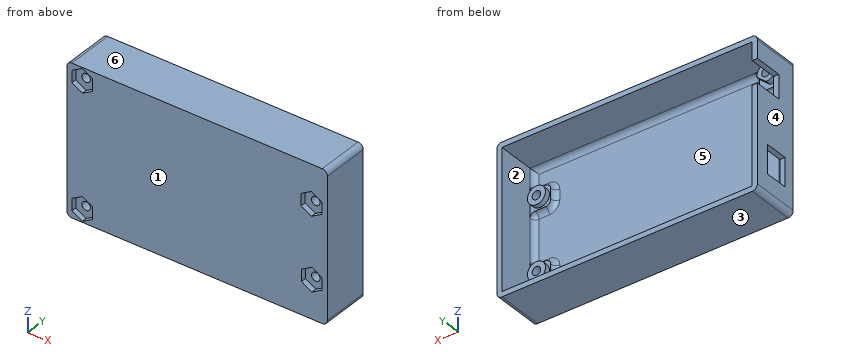
from build123d import *

# Parameters (mm, degrees)
SKETCH1_W           = 100.75
SKETCH1_H           = 57.75
SKETCH1_W_2         = 96.75
SKETCH1_H_2         = 53.75
SKETCH1_R           = 1.65
BOSS_EXTRUDE1_DEPTH = 2
SKETCH2_R           = 3.5
SKETCH2_R_2         = 1.65
BOSS_EXTRUDE2_DEPTH = 4
SKETCH3_W           = 100.75
SKETCH3_H           = 57.75
SKETCH3_W_2         = 96.75
SKETCH3_H_2         = 53.75
BOSS_EXTRUDE3_DEPTH = 16.4
FILLET1_R           = 2
SKETCH5_W           = 8
SKETCH5_H           = 8
SKETCH5_R           = 1.65
BOSS_EXTRUDE4_DEPTH = 2
FILLET3_R           = 2
FILLET4_R           = 2
SKETCH6_W           = 9.2
SKETCH6_H           = 11
SKETCH6_W_2         = 8
SKETCH6_H_2         = 2.6
CUT_EXTRUDE2_DEPTH  = 2
CUT_EXTRUDE3_DEPTH  = 2


with BuildPart() as part:
    # Sketch1 → Boss-Extrude1 (new body)
    # profile 1 of 2: a face of its own
    with BuildSketch(Plane(origin=(0, 0, 0), x_dir=(1, 0, 0), z_dir=(0, 1, 0))):
        with Locations((0.125, -0.125)):
            Rectangle(SKETCH1_W, SKETCH1_H)
        with Locations((0.125, -0.125)):
            Rectangle(SKETCH1_W_2, SKETCH1_H_2, mode=Mode.SUBTRACT)
    # profile 2 of 2: a face of its own
    with BuildSketch(Plane(origin=(0, 0, 0), x_dir=(1, 0, 0), z_dir=(0, 1, 0))):
        with Locations((0.125, -0.125)):
            Rectangle(SKETCH1_W_2, SKETCH1_H_2)
        with Locations(Location((-44.25, -24, 0), (0, 0, 270))):
            Circle(SKETCH1_R, mode=Mode.SUBTRACT)
        with Locations(Location((-44.25, 23.75, 0), (0, 0, 270))):
            Circle(SKETCH1_R, mode=Mode.SUBTRACT)
        with Locations(Location((44.5, 14, 0), (0, 0, 270))):
            Circle(SKETCH1_R, mode=Mode.SUBTRACT)
        with Locations(Location((44.5, -14.25, 0), (0, 0, 270))):
            Circle(SKETCH1_R, mode=Mode.SUBTRACT)
    extrude(amount=BOSS_EXTRUDE1_DEPTH)

    # Sketch2 → Boss-Extrude2 (add)
    # profile 1 of 4: a face of its own
    with BuildSketch(Plane(origin=(0, 2, 0), x_dir=(1, 0, 0), z_dir=(0, 1, 0))):
        with Locations(Location((44.5, 14, 0), (0, 0, 270))):
            Circle(SKETCH2_R)
        with Locations(Location((44.5, 14, 0), (0, 0, 270))):
            Circle(SKETCH2_R_2, mode=Mode.SUBTRACT)
    # profile 2 of 4: a face of its own
    with BuildSketch(Plane(origin=(0, 2, 0), x_dir=(1, 0, 0), z_dir=(0, 1, 0))):
        with Locations(Location((44.5, -14.25, 0), (0, 0, 270))):
            Circle(SKETCH2_R)
        with Locations(Location((44.5, -14.25, 0), (0, 0, 270))):
            Circle(SKETCH2_R_2, mode=Mode.SUBTRACT)
    # profile 3 of 4: a face of its own
    with BuildSketch(Plane(origin=(0, 2, 0), x_dir=(1, 0, 0), z_dir=(0, 1, 0))):
        with BuildLine():
            Line((-44.303434376, -20.500407914), (-40.787920243, -23.486187041))
            ThreePointArc((-40.787920243, -23.486187041), (-41.085130973, -25.494524687), (-42.447224362, -27))
            Line((-42.447224362, -27), (-46.052775638, -27))
            ThreePointArc((-46.052775638, -27), (-47.629726797, -23.090358985), (-44.303434376, -20.500407914))
        make_face()
        with Locations(Location((-44.25, -24, 0), (0, 0, 270))):
            Circle(SKETCH2_R_2, mode=Mode.SUBTRACT)
    # profile 4 of 4: a face of its own
    with BuildSketch(Plane(origin=(0, 2, 0), x_dir=(1, 0, 0), z_dir=(0, 1, 0))):
        with BuildLine():
            Line((-46.052775638, 26.75), (-42.447224362, 26.75))
            ThreePointArc((-42.447224362, 26.75), (-44.25, 20.25), (-46.052775638, 26.75))
        make_face()
        with Locations(Location((-44.25, 23.75, 0), (0, 0, 270))):
            Circle(SKETCH2_R_2, mode=Mode.SUBTRACT)
    extrude(amount=BOSS_EXTRUDE2_DEPTH)

    # Sketch3 → Boss-Extrude3 (add)
    with BuildSketch(Plane(origin=(0, 2, 0), x_dir=(1, 0, 0), z_dir=(0, 1, 0))):
        with Locations((0.125, -0.125)):
            Rectangle(SKETCH3_W, SKETCH3_H)
        with Locations((0.125, -0.125)):
            Rectangle(SKETCH3_W_2, SKETCH3_H_2, mode=Mode.SUBTRACT)
    extrude(amount=BOSS_EXTRUDE3_DEPTH)

    # Fillet1
    fillet1_edges = [part.edges().sort_by_distance(p)[0] for p in [
        (50.5, 9.2, 29),
        (-50.25, 9.2, 29),
        (-50.25, 9.2, -28.75),
        (50.5, 9.2, -28.75),
    ]]
    fillet(fillet1_edges, radius=FILLET1_R)

    # Sketch5 → Boss-Extrude4 (add)
    # profile 1 of 4: a face of its own
    with BuildSketch(Plane(origin=(0, 2, 0), x_dir=(1, 0, 0), z_dir=(0, 1, 0))):
        with Locations((44.5, 14)):
            Rectangle(SKETCH5_W, SKETCH5_H)
        with Locations(Location((44.5, 14, 0), (0, 0, 270))):
            Circle(SKETCH5_R, mode=Mode.SUBTRACT)
    # profile 2 of 4: a face of its own
    with BuildSketch(Plane(origin=(0, 2, 0), x_dir=(1, 0, 0), z_dir=(0, 1, 0))):
        with Locations((44.5, -14.25)):
            Rectangle(SKETCH5_W, SKETCH5_H)
        with Locations(Location((44.5, -14.25, 0), (0, 0, 270))):
            Circle(SKETCH5_R, mode=Mode.SUBTRACT)
    # profile 3 of 4: a face of its own
    with BuildSketch(Plane(origin=(0, 2, 0), x_dir=(1, 0, 0), z_dir=(0, 1, 0))):
        with Locations((-44.25, -23)):
            Rectangle(SKETCH5_W, SKETCH5_H)
        with Locations(Location((-44.25, -24, 0), (0, 0, 270))):
            Circle(SKETCH5_R, mode=Mode.SUBTRACT)
    # profile 4 of 4: a face of its own
    with BuildSketch(Plane(origin=(0, 2, 0), x_dir=(1, 0, 0), z_dir=(0, 1, 0))):
        with Locations((-44.25, 22.75)):
            Rectangle(SKETCH5_W, SKETCH5_H)
        with Locations(Location((-44.25, 23.75, 0), (0, 0, 270))):
            Circle(SKETCH5_R, mode=Mode.SUBTRACT)
    extrude(amount=BOSS_EXTRUDE4_DEPTH)

    # Fillet3
    fillet3_edges = [part.edges().sort_by_distance(p)[0] for p in [
        (40.5, 3, -18),
        (40.5, 3, -10),
        (48.5, 3, -10),
        (48.5, 3, -18),
        (40.5, 3, 10.25),
        (40.5, 3, 18.25),
        (48.5, 3, 18.25),
        (48.5, 3, 10.25),
        (-48.25, 3, 19),
        (-40.25, 3, 27),
        (-40.25, 3, 19),
        (-40.25, 3, -26.75),
        (-48.25, 3, -18.75),
        (-40.25, 3, -18.75),
    ]]
    fillet(fillet3_edges, radius=FILLET3_R)

    # Fillet4
    fillet4_edges = [part.edges().sort_by_distance(p)[0] for p in [
        (48.5, 2, -23.375),
        (47.914213562, 2, -18.585786438),
        (44.5, 2, -18),
        (41.085786438, 2, -17.414213562),
        (48.5, 2, 23.625),
        (47.914213562, 2, 18.835786438),
        (44.5, 2, 18.25),
        (41.085786438, 2, 17.664213562),
        (40.5, 2, 14.25),
        (41.085786438, 2, 10.835786438),
        (44.5, 2, 10.25),
        (47.914213562, 2, 9.664213562),
        (48.5, 2, 0.125),
        (47.914213562, 2, -9.414213562),
        (44.5, 2, -10),
        (41.085786438, 2, -10.585786438),
        (5.125, 2, 27),
        (-39.664213562, 2, 26.414213562),
        (-40.25, 2, 23),
        (-40.835786438, 2, 19.585786438),
        (5.125, 2, -26.75),
        (-39.664213562, 2, -26.164213562),
        (-40.25, 2, -22.75),
        (-40.835786438, 2, -19.335786438),
        (-44.25, 2, -18.75),
        (-47.664213562, 2, -18.164213562),
        (-48.25, 2, 0.125),
        (-47.664213562, 2, 18.414213562),
        (40.5, 2, -14),
        (-44.25, 2, 19),
    ]]
    fillet(fillet4_edges, radius=FILLET4_R - 0.0001)  # a hair under: the kernel refuses the full size

    # Sketch6 → Cut-Extrude2 (cut)
    with BuildSketch(Plane.ZY.offset(50.25)):
        with Locations((15.4, 12.9)):
            Rectangle(SKETCH6_W, SKETCH6_H)
        Polygon((-18.75, 7.4), (-20.25, 7.4), (-20.25, 4.2), (-9.25, 4.2), (-9.25, 7.4), (-10.75, 7.4), align=None)
        Polygon((-20.25, 13.2), (-20.25, 7.4), (-18.75, 7.4), (-18.75, 10), (-10.75, 10), (-10.75, 7.4), (-9.25, 7.4), (-9.25, 13.2), align=None)
        with Locations((-14.75, 8.7)):
            Rectangle(SKETCH6_W_2, SKETCH6_H_2)
    extrude(amount=-CUT_EXTRUDE2_DEPTH, mode=Mode.SUBTRACT)

    # Sketch4 → Cut-Extrude3 (cut)
    with BuildSketch(Plane.XZ):
        Polygon((40.5, -11.690598923), (40.5, -16.309401077), (44.5, -18.618802154), (48.5, -16.309401077), (48.5, -11.690598923), (44.5, -9.381197846), align=None)
        Polygon((40.355047504, 11.886928072), (44.355047504, 9.577526995), (48.355047504, 11.886928072), (48.355047504, 16.505730226), (44.355047504, 18.815131302), (40.355047504, 16.505730226), align=None)
        Polygon((-48.25, 26.309401077), (-48.25, 21.690598923), (-44.25, 19.381197846), (-40.25, 21.690598923), (-40.25, 26.309401077), (-44.25, 28.618802154), align=None)
        Polygon((-44.25, -19.131197846), (-48.25, -21.440598923), (-48.25, -26.059401077), (-44.25, -28.368802154), (-40.25, -26.059401077), (-40.25, -21.440598923), align=None)
    extrude(amount=-CUT_EXTRUDE3_DEPTH, mode=Mode.SUBTRACT)


solid = part.part
Build history of the part. All positions in model axes, mm. Face numbers are marked on the shaded views. A direction names the side the tool comes from. Give positions to 0.01 mm unless a question says otherwise; leave off trailing zeros. Order: outer loops, then holes, each group sorted by start corner. A loop starts at its lowest first (then second) coordinate and runs counter-clockwise, first axis right, second up. Notation, with made-up numbers: M 20,49.25 L 31,49.25 A21 ccw 31,65.25 Z; hole C -22,48 d6. An arc over 180 degrees is marked long. Use one line per item in the form item = value.
Q1. Slice it at C-C, the plane x = -13. Write the cut outline in (y, z).
Conclusion:
outline = M 0,-28.75 L 18.4,-28.75 L 18.4,-26.75 L 4,-26.75 A2 cw 2,-24.75 L 2,25 A2 cw 4,27 L 18.4,27 L 18.4,29 L 0,29 Z
Q2. Pin check, flat tips, straight feed: P1, Ø4, axis at x = -21.5, z = -10.5, coming from the +Y side; P2, Ø1, axis at x = -49, y = 11, coming from the +Z side; P3, Ø3.5, axis at x = 44.5, z = 15.5, coming from the +Y side. Stop position of each tip, or through.
Conclusion:
P1 = 2
P2 = 28.98
P3 = 6
Q3. Pull direction Z, two halves, no side cores. Call the marked faces 3, 4, 5 and 6: released by +Z, released by -Z, zero draft, split by the parting line, or undercut.
Conclusion:
face_3 = released by -Z
face_4 = zero draft
face_5 = undercut
face_6 = released by +Z
Q4. Which spindle directions (+Z, -Z, +X, -X, +Y, -Y) get a long thin tool onto all of the face, cutting with end or side? Do the marked faces 1 and 2. Say none if no direction does.
Conclusion:
face_1 = +Z, -Z, +X, -X, -Y
face_2 = +Y
Q5. Slice it at D-D, the plane y = 14.75. Write the cut outline in (x, z), and give its area (3 significant figures).
Conclusion:
outline = M -50.25,-26.75 A2 ccw -48.25,-28.75 L 48.5,-28.75 A2 ccw 50.5,-26.75 L 50.5,27 A2 ccw 48.5,29 L -48.25,29 A2 ccw -50.25,27 L -50.25,20 L -48.25,20 L -48.25,27 L 48.5,27 L 48.5,-26.75 L -48.25,-26.75 L -48.25,10.8 L -50.25,10.8 Z
area = 596 mm2
Q6. Slice it at A-A, the plane z = -14. State how many separate pieces and enclosed holes the cut face has, and give its area (3 significant figures).
Conclusion:
separate_pieces = 3
enclosed_holes = 0
area = 252 mm2
Q7. Wall check: probe 1 along X at (y, z) = (4.5, -23.75); probe 2 along X at (y, z) = (5.1, 14.25); probe 3 along Z at (x, y) = (44.5, 4.55). Give the ranges that are in metal, low to high.
Conclusion:
probe_1 = -50.25 to -48.25, -47.75 to -45.9, -42.6 to -40.75, 48.5 to 50.5
probe_2 = -50.25 to -48.25, 41 to 42.85, 46.15 to 48, 48.5 to 50.5
probe_3 = -28.75 to -26.75, -17.5 to -15.65, -12.35 to -10.5, 10.75 to 12.6, 15.9 to 17.75, 27 to 29
